The listing builds one solid part. Answer for the finished solid, in the listing's coordinates (mm). Face numbers are marked on the shaded views. A direction names the side the tool comes from. Coordinates: 2 decimals unless noted, no trailing zeros. Loops run counter-clockwise (first coordinate to the right, second up) from the corner with the lowest first, then second, coordinate; pieces in that order, holes last. Notation, with made-up numbers: (-32.5, 83) -> (19.5, 83) arc R33 ccw to (19.5, 117) -> close; hole circle Ø1 at (18, 4). An arc over 180 degrees is marked (long way). Answer in a Markdown table with one row per item.
```python
from build123d import *

# Parameters (mm, degrees)
F1_DEPTH = 50
F0_R     = 3.125
F2_DEPTH = 7.5
F0_R_2   = 1.625
F3_DEPTH = 5


# Not quite as in the source:
# - a fillet or chamfer that OpenCascade refuses, or shapes differently, is made with other operations: its cross-section is extruded or revolved along the edge and cut away or added


with BuildPart() as f1:
    # F0 (on Top) → F1 (new body)
    with BuildSketch(Plane.XY):
        with BuildLine():
            ThreePointArc((0, -7.5), (5.3033008589, -5.3033008589), (7.5, 0))
            ThreePointArc((7.5, 0), (5.3033008589, 5.3033008589), (0, 7.5))
            ThreePointArc((0, 7.5), (-7.5, 0), (0, -7.5))
        make_face()
    extrude(amount=F1_DEPTH)

    # F0 (on Top) → F2 (join)
    with BuildSketch(Plane.XY):
        with BuildLine():
            ThreePointArc((0, 7.5), (5.3033008589, 5.3033008589), (7.5, 0))
            ThreePointArc((7.5, 0), (5.3033008589, -5.3033008589), (0, -7.5))
            Line((0, -7.5), (12.5, -7.5))
            ThreePointArc((12.5, -7.5), (17.8033008589, -5.3033008589), (20, 0))
            ThreePointArc((20, 0), (17.8033008589, 5.3033008589), (12.5, 7.5))
            Line((12.5, 7.5), (0, 7.5))
        make_face()
        with Locations((12.5, 0)):
            Circle(F0_R, mode=Mode.SUBTRACT)
    extrude(amount=F2_DEPTH)

    # F0 (on Top) → F3 (join)
    with BuildSketch(Plane.XY):
        with Locations((12.5, 0)):
            Circle(F0_R)
        with Locations((12.5, 0)):
            Circle(F0_R_2, mode=Mode.SUBTRACT)
    extrude(amount=F3_DEPTH)

    # F4: chamfer of 5 on 1 edges, made by hand

    # F4_s1 → F4_t2 (revolve, cut)
    with BuildSketch(Plane.YZ):
        Polygon((-7.5, 45), (-2.5, 50), (-7.5, 50), align=None)
    revolve(axis=Axis((0, 0, 50), (0, 0, -1)), mode=Mode.SUBTRACT)


solid = f1.part
```
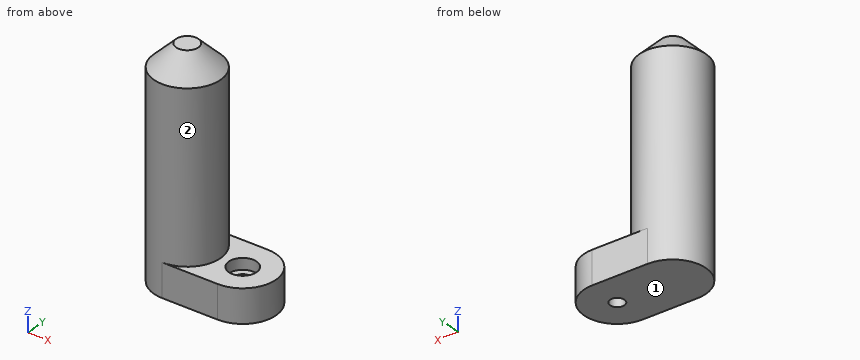
Item 1: A cutting plane is placed at A-A, the plane y = 0. Determine the outline of the cut face in (x, z) (3 decimals), plus the area to 3 significant figures.
Findings below:
| item | result |
|---|---|
| outline | (-7.5, 0) -> (10.875, 0) -> (10.875, 5) -> (9.375, 5) -> (9.375, 7.5) -> (7.5, 7.5) -> (7.5, 45) -> (2.5, 50) -> (-2.5, 50) -> (-7.5, 45) -> close; (14.125, 0) -> (20, 0) -> (20, 7.5) -> (15.625, 7.5) -> (15.625, 5) -> (14.125, 5) -> close |
| area | 787 mm2 |
Item 2: Flat-ended cylindrical pins translate along their axes: pin 1 Ø5.5 at (x, y) = (12.5, 0) entering from +Z; pin 2 Ø4 at (y, z) = (1, 33) entering from +X; pin 3 Ø5 at (x, y) = (11, 1) entering from +Z. Find the tip coordinate at first contact, or state that the pin passes through.
Findings below:
| item | result |
|---|---|
| pin 1 | stops at z = 5 |
| pin 2 | stops at x = 7.5 |
| pin 3 | stops at z = 7.5 |
Item 3: A cutting plane is placed at B-B, the plane z = 21.5. Determine the outline of the cut face in (x, y), plus the area to 3 significant figures.
Findings below:
| item | result |
|---|---|
| outline | circle Ø15 at (0, 0) |
| area | 177 mm2 |
Item 4: A tool of negligible diameter and unlimited length cuts with its end or side. For the marked faces 1 and 2, from which of +Z, -Z, +X, -X, +Y, -Y can it reach the whole face along a straight path? Write none if from no direction.
Findings below:
| item | result |
|---|---|
| face 1 | -Z, +X, -X, +Y, -Y |
| face 2 | +Z |
Item 5: Find the intervals of material crossed by probe 1 along Y at (x, z) = (12.5, 5.9) (3 decimals); probe 2 along Y at (x, z) = (12.5, 3.3) (3 decimals); probe 3 along X at (y, z) = (-0.25, 42), in increasing order.
Findings below:
| item | result |
|---|---|
| probe 1 | y = -7.5 to -3.125, 3.125 to 7.5 |
| probe 2 | y = -7.5 to -1.625, 1.625 to 7.5 |
| probe 3 | x = -7.5 to 7.5 |
